```python
from build123d import *

# Parameters (mm, degrees)
EXTRUDE_1_DEPTH     = 2
SKETCH_2_R          = 1.45
CUT_EXTRUDE_1_DEPTH = 58.043842788
FILLET_1_R          = 2


with BuildPart() as part:
    # 草图1 → 凸台-拉伸1 (new body)
    with BuildSketch(Plane.XY):
        Polygon((0, 0), (7.5, 30), (27.5, 30), (35, 0), (35, -15), (27.5, -45), (7.5, -45), (0, -15), align=None)
    extrude(amount=EXTRUDE_1_DEPTH)

    # 草图2 → 切除-拉伸1 (cut, through all)
    with BuildSketch(Plane.XY.offset(2)):
        with Locations((7.5, -7.5)):
            Circle(SKETCH_2_R)
        with Locations(Location((27.5, -7.5, 0), (0, 0, 180))):
            Circle(SKETCH_2_R)
        with BuildLine():
            Line((19, 25), (19, 5))
            ThreePointArc((19, 5), (17.5, 3.5), (16, 5))
            Line((16, 5), (16, 25))
            ThreePointArc((16, 25), (17.5, 26.5), (19, 25))
        make_face()
        with BuildLine():
            Line((19, -40), (19, -20))
            ThreePointArc((19, -20), (17.5, -18.5), (16, -20))
            Line((16, -20), (16, -40))
            ThreePointArc((16, -40), (17.5, -41.5), (19, -40))
        make_face()
    extrude(amount=-CUT_EXTRUDE_1_DEPTH, mode=Mode.SUBTRACT)

    # 圆角1
    fillet_1_edges = [part.edges().sort_by_distance(p)[0] for p in [
        (0, 0, 1),
        (7.5, 30, 1),
        (27.5, 30, 1),
        (35, 0, 1),
        (35, -15, 1),
        (27.5, -45, 1),
        (7.5, -45, 1),
        (0, -15, 1),
    ]]
    fillet(fillet_1_edges, radius=FILLET_1_R)


solid = part.part
```
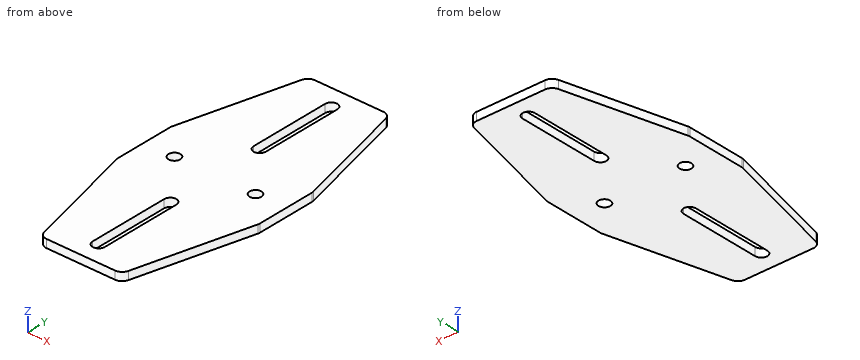
CAD build for the part. Positions are in the model's coordinates, mm. Round coordinates to 2 decimals unless told otherwise and drop trailing zeros. Order: outer loops, then holes, each group sorted by start corner. A loop starts at its lowest first (then second) coordinate and runs counter-clockwise, first axis right, second up. Notation, with made-up numbers: (-3, 43.5) -> (21, 43.5) arc R16 cw to (21, 59.5) -> close; hole circle Ø6 at (85.25, 59.5). An arc over 180 degrees is marked (long way). One line per question, with ' | ' between items.
Q1. Drop flat-ended pins along their axis: pin 1 (0.6 mm diameter, centred on y = -28.5, z = 1, fed in from -X); pin 2 (0.6 mm diameter, centred on y = 10.5, z = 1, fed in from +X); pin 3 (1 mm diameter, centred on y = 16.5, z = 0.5, fed in from -X). Give the stop position or say it passes through.
Completed:
pin 1: stops at x = 3.3 | pin 2: stops at x = 32.45 | pin 3: stops at x = 4
Q2. Slice it at A-A (x = 17.5). Write the cut outline in (y, z), then the cut area to 3 significant figures.
Completed:
outline: (-45, 0) -> (-41.5, 0) -> (-41.5, 2) -> (-45, 2) -> close; (-18.5, 0) -> (3.5, 0) -> (3.5, 2) -> (-18.5, 2) -> close; (26.5, 0) -> (30, 0) -> (30, 2) -> (26.5, 2) -> close | area: 58.0 mm^2
Q3. Probe probe 1 along Y at (x, z) = (17.5, 1.25); probe 2 along X at (y, z) = (20, 0.5); probe 3 along X at (y, z) = (-7, 1.9). List the from-to ranges inside material, lowest first.
Completed:
probe 1: y = -45 to -41.5, -18.5 to 3.5, 26.5 to 30 | probe 2: x = 5 to 16, 19 to 30 | probe 3: x = 0 to 6.14, 8.86 to 26.14, 28.86 to 35
Q4. Slice it at C-C (z = 0.85). Write the cut outline in (x, y).
Completed:
outline: (0, -14.75) arc R2 ccw to (0.06, -15.24) -> (7.12, -43.49) arc R2 ccw to (9.06, -45) -> (25.94, -45) arc R2 ccw to (27.88, -43.49) -> (34.94, -15.24) arc R2 ccw to (35, -14.75) -> (35, -0.25) arc R2 ccw to (34.94, 0.24) -> (27.88, 28.49) arc R2 ccw to (25.94, 30) -> (9.06, 30) arc R2 ccw to (7.12, 28.49) -> (0.06, 0.24) arc R2 ccw to (0, -0.25) -> close; hole circle Ø2.9 at (7.5, -7.5); hole (16, -40) arc R1.5 ccw to (19, -40) -> (19, -20) arc R1.5 ccw to (16, -20) -> close; hole (16, 5) arc R1.5 ccw to (19, 5) -> (19, 25) arc R1.5 ccw to (16, 25) -> close; hole circle Ø2.9 at (27.5, -7.5)
Q5. Slice it at D-D (y = -25). Write the cut outline in (x, z), then the cut area to 3 significant figures.
Completed:
outline: (2.5, 0) -> (16, 0) -> (16, 2) -> (2.5, 2) -> close; (19, 0) -> (32.5, 0) -> (32.5, 2) -> (19, 2) -> close | area: 54.0 mm^2
Q6. Slice it at B-B (y = -7.5). Write the cut outline in (x, z).
Completed:
outline: (0, 0) -> (6.05, 0) -> (6.05, 2) -> (0, 2) -> close; (8.95, 0) -> (26.05, 0) -> (26.05, 2) -> (8.95, 2) -> close; (28.95, 0) -> (35, 0) -> (35, 2) -> (28.95, 2) -> close
